Check sheet for the modelled part. Datum: model origin and axes. Units: mm. A direction names the side the tool comes from. Give positions to 0.01 mm unless a question says otherwise; leave off trailing zeros. Write each loop counter-clockwise with the first axis right and the second up, starting at its lowest first coordinate (ties: lowest second). Pieces come first, ordered by that corner, then holes. Notation, with made-up numbers: M 33,34 L 72,34 A18 ccw 72,44 Z; hole C -2.75,84 d4. An arc over 180 degrees is marked long. Write item = value, one per line. Start each with the question number.
1) Go/stop test with flat-tipped pins: pin 1 (14.5 mm diameter, centred on y = -6.5, z = -24, fed in from +X); pin 2 (3 mm diameter, centred on x = 15, y = -6.5, fed in from -Z); pin 3 (5 mm diameter, centred on x = 8, y = -15.5, fed in from +Z). Record where each tip stops, or that it passes through.
2) Mould release check, pull along X, two halves, no side actions. Record for faces 1 (the flat face through (5.291, -6, 27)), 2 (the flat face through (19.744, -6, 15)), 3 (the flat face through (0, 0, 1)): released by +X, released by -X, zero draft, split by the parting line, or undercut.
3) Cross-section at C-C, the plane x = 0. Record the cut outline in (y, z).
4) Scan lines: line 1 along X through (y, z) = (-11, 28); line 2 along Y through (x, z) = (-10.5, 31); line 3 along Z through (x, y) = (-17, -37). Record each from-to range of solid material in increasing order. Write a range as [from, to].
5) Access from +Z, -Z, +X, -X, +Y, -Y to the whole of each face (thin tool, end or side, straight path). Record for faces 4 (the flat face through (0, -31, -21.165)), 5 (the flat face through (15, -18.288, -28)), 6 (the flat face through (-5.291, -6, 27)).
6) Cross-section at D-D, the plane z = -10.5. Record the cut outline in (x, y), plus the area to 3 significant figures.
7) Cross-section at A-A, the plane z = 25.5. Record the cut outline in (x, y).
8) Cross-section at B-B, the plane x = 14. Record the cut outline in (y, z).
```python
from build123d import *

# Parameters (mm, degrees)
F0_W     = 39.4888110459
F0_H     = 71.7479661107
F1_DEPTH = 12.7
F2_W     = 39.4888110459
F2_H     = 14.7085804492
F3_DEPTH = 38.1
F5_DEPTH = 25.4
F7_DEPTH = 25.4
F8_W     = 10.5819702148
F8_H     = 30.0025250763
F9_DEPTH = 18.288


with BuildPart() as f1:
    # F0 (on Front) → F1 (new body)
    with BuildSketch(Plane.XZ):
        Rectangle(F0_W, F0_H)
    extrude(amount=F1_DEPTH)

    # F2 (on face) → F3 (join)
    with BuildSketch(Plane.XZ.offset(12.7)):
        with Locations((0, -28.5196928307)):
            Rectangle(F2_W, F2_H)
    extrude(amount=F3_DEPTH)

    # F4 (on face) → F5 (cut)
    with BuildSketch(Plane.XZ.offset(12.7)):
        with BuildLine():
            Line((-5.2909860387, 53.4245613962), (-5.2909860387, 18.3234047145))
            Line((-5.2909860387, 18.3234047145), (-5.2212785764, 18.3234047145))
            ThreePointArc((-5.2212785764, 18.3234047145), (0, 13.1021261381), (5.2212785764, 18.3234047145))
            Line((5.2212785764, 18.3234047145), (5.2909860387, 18.3234047145))
            Line((5.2909860387, 18.3234047145), (5.2909860387, 53.4245613962))
            Line((5.2909860387, 53.4245613962), (-5.2909860387, 53.4245613962))
        make_face()
    extrude(amount=-F5_DEPTH, mode=Mode.SUBTRACT)

    # F6 (on face) → F7 (cut)
    with BuildSketch(Plane.XY.offset(-21.1654026061)):
        with BuildLine():
            ThreePointArc((-1.976119183, -50.8), (-14.4143084854, -44.6129399446), (-19.6615021384, -31.75))
            Line((-19.6615021384, -31.75), (-19.7444055229, -31.75))
            Line((-19.7444055229, -31.75), (-19.7444055229, -50.8))
            Line((-19.7444055229, -50.8), (-1.976119183, -50.8))
        make_face()
        with BuildLine():
            Line((19.7444055229, -31.75), (19.6615021384, -31.75))
            ThreePointArc((19.6615021384, -31.75), (14.4143084854, -44.6129399446), (1.976119183, -50.8))
            Line((1.976119183, -50.8), (19.7444055229, -50.8))
            Line((19.7444055229, -50.8), (19.7444055229, -31.75))
        make_face()
    extrude(amount=-F7_DEPTH, mode=Mode.SUBTRACT)

    # F8 (on face) → F9 (cut)
    with BuildSketch(Plane(origin=(0, 0, 0), x_dir=(-1, 0, 0), z_dir=(0, 1, 0))):
        with Locations((-14.4534204155, -20.8727205172)):
            Rectangle(F8_W, F8_H)
    extrude(amount=-F9_DEPTH, mode=Mode.SUBTRACT)


solid = f1.part
```
Reply:
q1.pin_1 = 9.16
q1.pin_2 = -5.87
q1.pin_3 = -21.17
q2.face_1 = undercut
q2.face_2 = released by +X
q2.face_3 = zero draft
q3.outline = M -50.8,-35.87 L 0,-35.87 L 0,13.1 L -12.7,13.1 L -12.7,-21.17 L -50.8,-21.17 Z
q4.line_1 = [-19.74, -5.29], [5.29, 19.74]
q4.line_2 = [-12.7, 0]
q4.line_3 = [-35.87, -21.17]
q5.face_4 = +Z, +X, -X, -Y
q5.face_5 = +Z, -Z, +X, +Y
q5.face_6 = +Z, +Y, -Y
q6.outline = M -19.74,-12.7 L 9.16,-12.7 L 9.16,0 L -19.74,0 Z
q6.area = 367 mm2
q7.outline = M -19.74,-12.7 L -5.29,-12.7 L -5.29,0 L -19.74,0 Z; M 5.29,-12.7 L 19.74,-12.7 L 19.74,0 L 5.29,0 Z
q8.outline = M -45.05,-35.87 L -18.29,-35.87 L -18.29,-21.17 L -45.05,-21.17 Z; M -12.7,-5.87 L 0,-5.87 L 0,35.87 L -12.7,35.87 Z
